from build123d import *

# Parameters (mm, degrees)
PAD_DEPTH           = 2
PAD001_DEPTH        = 3
PAD002_DEPTH        = 3.6
PAD003_DEPTH        = 5
SKETCH004_W         = 63
SKETCH004_H         = 17.5
POCKET_DEPTH        = 11.7
PAD004_DEPTH        = 18
HOLE_D              = 3.3
HOLE_DEPTH          = 24.00858
HOLE_CSINK_D        = 6
HOLE_CSINK_ANGLE    = 90
HOLE_TIPS_R         = 1.65
SKETCH010_R         = 1.75
POCKET001_DEPTH     = 5
HOLE001_D           = 3.3
HOLE001_DEPTH       = 24.00858
HOLE001_CSINK_D     = 6
HOLE001_CSINK_ANGLE = 90
HOLE001_TIPS_R      = 1.65
HOLE002_D           = 3.3
HOLE002_DEPTH       = 24.00858
HOLE002_CSINK_D     = 6
HOLE002_CSINK_ANGLE = 90
HOLE002_TIPS_R      = 1.65


with BuildPart() as part:
    # Sketch → Pad (new body)
    with BuildSketch(Plane.XY):
        Polygon((-31.5, 17.5), (31.5, 17.5), (31.5, -17.5), (15.54, -17.5), (15.54, 2.8e-05), (7.77, 13.458035), (-7.77, 13.458035), (-15.54, 0), (-15.54, -17.5), (-31.5, -17.5), align=None)
    extrude(amount=PAD_DEPTH)

    # Sketch001 (on Face12 of Pad) → Pad001 (join)
    with BuildSketch(Plane.XY.offset(2)):
        with BuildLine():
            ThreePointArc((10, 2.8e-05), (-1.4e-05, 10), (-10, 0))
            Line((-15.54, 0), (-10, 0))
            Line((-15.54, -17.5), (-15.54, 0))
            Line((-15.54, -17.5), (-31.5, -17.5))
            Line((-31.5, -17.5), (-31.5, 17.5))
            Line((-31.5, 17.5), (31.5, 17.5))
            Line((31.5, 17.5), (31.5, -17.5))
            Line((31.5, -17.5), (15.54, -17.5))
            Line((15.54, -17.5), (15.54, 2.8e-05))
            Line((10, 2.8e-05), (15.54, 2.8e-05))
        make_face()
    extrude(amount=PAD001_DEPTH)

    # Sketch002 (on Face20 of Pad001) → Pad002 (join)
    with BuildSketch(Plane.XY.offset(5)):
        Polygon((15.54, 0), (7.77, 13.458035), (-7.77, 13.458035), (-15.54, 0), (-15.54, -17.5), (-31.5, -17.5), (-31.5, 17.5), (31.5, 17.5), (31.5, -17.5), (15.54, -17.5), align=None)
    extrude(amount=PAD002_DEPTH)

    # Sketch003 (on Face31 of Pad002) → Pad003 (join)
    with BuildSketch(Plane.XY.offset(8.6)):
        with BuildLine():
            Line((-31.5, 17.5), (31.5, 17.5))
            Line((31.5, 17.5), (31.5, -17.5))
            Line((31.5, -17.5), (15.54, -17.5))
            Line((15.54, 0), (15.54, -17.5))
            Line((13, 0), (15.54, 0))
            ThreePointArc((13, 0), (0, 13), (-13, 0))
            Line((-15.54, 0), (-13, 0))
            Line((-15.54, 0), (-15.54, -17.5))
            Line((-15.54, -17.5), (-31.5, -17.5))
            Line((-31.5, -17.5), (-31.5, 17.5))
        make_face()
    extrude(amount=PAD003_DEPTH)

    # Sketch004 (on Face41 of Pad003) → Pocket (cut)
    with BuildSketch(Plane.XY.offset(13.6)):
        with Locations((0, -8.75)):
            Rectangle(SKETCH004_W, SKETCH004_H)
    extrude(amount=-POCKET_DEPTH, mode=Mode.SUBTRACT)

    # Sketch008 (on Face1 of Pocket) → Pad004 (join)
    with BuildSketch(Plane(origin=(0, 0, 0), x_dir=(1, 0, 0), z_dir=(0, 0, -1))):
        Polygon((-7.77, -13.458035), (7.77, -13.458035), (15.54, -2.8e-05), (18.54, 0), (8.23, -17.5), (-7.77, -17.5), (-18.54, 0), (-15.54, 0), align=None)
    extrude(amount=PAD004_DEPTH)

    # Hole
    with Locations(Plane(origin=(0, 17.5, 0), x_dir=(-1, 0, 0), z_dir=(0, 1, 0))):
        with Locations((0, -2.45), (-4.5, -10.45), (4.5, -10.45)):
            CounterSinkHole(HOLE_D / 2, HOLE_CSINK_D / 2, depth=HOLE_DEPTH, counter_sink_angle=HOLE_CSINK_ANGLE)

    # Hole tips → Hole tip 1 section 0
    with BuildSketch(Plane(origin=(0, -6.50858, 0), x_dir=(-1, 0, 0), z_dir=(0, 1, 0)), mode=Mode.PRIVATE) as hole_tip_1_s0:
        with Locations((0, -2.45)):
            Circle(HOLE_TIPS_R)
    loft([hole_tip_1_s0.sketch, Vertex(0, -7.5, -2.45)], mode=Mode.SUBTRACT)

    # Hole tips → Hole tip 2 section 0
    with BuildSketch(Plane(origin=(0, -6.50858, 0), x_dir=(-1, 0, 0), z_dir=(0, 1, 0)), mode=Mode.PRIVATE) as hole_tip_2_s0:
        with Locations((-4.5, -10.45)):
            Circle(HOLE_TIPS_R)
    loft([hole_tip_2_s0.sketch, Vertex(4.5, -7.5, -10.45)], mode=Mode.SUBTRACT)

    # Hole tips → Hole tip 3 section 0
    with BuildSketch(Plane(origin=(0, -6.50858, 0), x_dir=(-1, 0, 0), z_dir=(0, 1, 0)), mode=Mode.PRIVATE) as hole_tip_3_s0:
        with Locations((4.5, -10.45)):
            Circle(HOLE_TIPS_R)
    loft([hole_tip_3_s0.sketch, Vertex(-4.5, -7.5, -10.45)], mode=Mode.SUBTRACT)

    # Sketch010 (on Face32 of Hole) → Pocket001 (cut)
    with BuildSketch(Plane.XY.offset(1.9)):
        with Locations((-22.54, -10.7)):
            Circle(SKETCH010_R)
        with Locations((22.54, -10.7)):
            Circle(SKETCH010_R)
    extrude(amount=-POCKET001_DEPTH, mode=Mode.SUBTRACT)

    # Hole001
    with Locations(Plane.XY.offset(13.6)):
        with Locations((-22.54, 10.7), (22.54, 10.7)):
            CounterSinkHole(HOLE001_D / 2, HOLE001_CSINK_D / 2, depth=HOLE001_DEPTH, counter_sink_angle=HOLE001_CSINK_ANGLE)

    # Hole001 tips → Hole001 tip 1 section 0
    with BuildSketch(Plane.XY.offset(-10.40858), mode=Mode.PRIVATE) as hole001_tip_1_s0:
        with Locations((-22.54, 10.7)):
            Circle(HOLE001_TIPS_R)
    loft([hole001_tip_1_s0.sketch, Vertex(-22.54, 10.7, -11.4)], mode=Mode.SUBTRACT)

    # Hole001 tips → Hole001 tip 2 section 0
    with BuildSketch(Plane.XY.offset(-10.40858), mode=Mode.PRIVATE) as hole001_tip_2_s0:
        with Locations((22.54, 10.7)):
            Circle(HOLE001_TIPS_R)
    loft([hole001_tip_2_s0.sketch, Vertex(22.54, 10.7, -11.4)], mode=Mode.SUBTRACT)

    # Hole002
    with Locations(Plane(origin=(0, 17.5, 0), x_dir=(-1, 0, 0), z_dir=(0, 1, 0))):
        with Locations((-27.5, 5.7), (27.5, 5.7)):
            CounterSinkHole(HOLE002_D / 2, HOLE002_CSINK_D / 2, depth=HOLE002_DEPTH, counter_sink_angle=HOLE002_CSINK_ANGLE)

    # Hole002 tips → Hole002 tip 1 section 0
    with BuildSketch(Plane(origin=(0, -6.50858, 0), x_dir=(-1, 0, 0), z_dir=(0, 1, 0)), mode=Mode.PRIVATE) as hole002_tip_1_s0:
        with Locations((-27.5, 5.7)):
            Circle(HOLE002_TIPS_R)
    loft([hole002_tip_1_s0.sketch, Vertex(27.5, -7.5, 5.7)], mode=Mode.SUBTRACT)

    # Hole002 tips → Hole002 tip 2 section 0
    with BuildSketch(Plane(origin=(0, -6.50858, 0), x_dir=(-1, 0, 0), z_dir=(0, 1, 0)), mode=Mode.PRIVATE) as hole002_tip_2_s0:
        with Locations((27.5, 5.7)):
            Circle(HOLE002_TIPS_R)
    loft([hole002_tip_2_s0.sketch, Vertex(-27.5, -7.5, 5.7)], mode=Mode.SUBTRACT)


solid = part.part
Input: part model. Units: mm. Frame: model coordinates. A direction names the side the tool comes from. Give positions to 0.01 mm unless a question says otherwise; leave off trailing zeros. Order: outer loops, then holes, each group sorted by start corner. A loop starts at its lowest first (then second) coordinate and runs counter-clockwise, first axis right, second up. Notation, with made-up numbers: (77.5, 39.25) - (92.5, 39.25) arc R22 cw to (92.5, 60.25) - close; hole circle Ø10 at (26, 9.25). An arc over 180 degrees is marked (long way). Answer as a JSON object with one key per item and string values. Group by question number.
Q1. Cut plane B-B, the plane y = -2.5. Output: boundary loops of the cut face in (x, z), then the cut area to 3 significant figures.
Q2. Cut plane C-C, the plane x = -22.54. Output: boundary loops of the cut face in (y, z), then the cut area to 3 significant figures.
Q3. Mould query, pull axis Z, two halves, no side actions, for faces 4 (the face through (0, 15, 13.6)), 5 (the face through (-31.5, 8, 7)), 6 (the face through (0, 13.458, 7)). Classes: pulls with the +Z half, pulls with the -Z half, needs draft (parallel to the pull), parting line crosses it, or undercut.
Q4. Set-up query: faces 1 (the face through (15.54, -9, 1)), 2 (the face through (11.601, 6.823, -7.86)), 3 (the face through (0, 13, 11)). Return all of +Z, -Z, +X, -X, +Y, -Y with unobstructed straight access to the full face (end or side cutting, diameter ignored); none if empty.
Q5. Cut plane A-A, the plane z = 5.7. Output: boundary loops of the cut face in (x, y).
Q6. Line query: probe 1 along Y at (x, z) = (-22.54, 0.5); probe 2 along Z at (x, y) = (-14, 2.5); probe 3 along Y at (x, z) = (22.54, 3.5). Output: solid intervals per line, ascending.
Q7. Cut plane D-D, the plane y = -10.7. Output: boundary loops of the cut face in (x, z).
Q8. First-contact query: pin 1 Ø4 at (x, y) = (-22.54, -10.7) entering from -Z; pin 2 Ø2.5 at (x, z) = (16.5, -7) entering from -Y; pin 3 Ø4 at (x, y) = (0.5, 9.5) entering from -Z; pin 4 Ø13 at (x, z) = (-21.5, 8) entering from -Y. Flat tips, straight axial feed; report the tip coordinate or a pass-through.
Results:
{
 "1": {"outline": "(-31.5, 0) - (-15.54, 0) - (-15.54, 1.9) - (-31.5, 1.9) - close; (15.54, 0) - (31.5, 0) - (31.5, 1.9) - (15.54, 1.9) - close", "area": "60.6 mm^2"},
 "2": {"outline": "(-17.5, 0) - (-12.45, 0) - (-12.45, 1.9) - (-17.5, 1.9) - close; (-8.95, 0) - (9.05, 0) - (9.05, 12.25) - (7.7, 13.6) - (0, 13.6) - (0, 1.9) - (-8.95, 1.9) - close; (12.35, 0) - (17.5, 0) - (17.5, 13.6) - (13.7, 13.6) - (12.35, 12.25) - close", "area": "218 mm^2"},
 "3": {"face 4": "pulls with the +Z half", "face 5": "needs draft", "face 6": "undercut"},
 "4": {"face 1": "+Z, -Z, -Y", "face 2": "-Z, -Y", "face 3": "+Z, -Y"},
 "5": {"outline": "(-31.5, 0) - (-29.15, 0) - (-29.15, 16.15) - (-30.5, 17.5) - (-31.5, 17.5) - close; (-25.85, 0) - (-15.54, 0) - (-7.77, 13.46) - (7.77, 13.46) - (15.54, 0) - (25.85, 0) - (25.85, 16.15) - (24.5, 17.5) - (-24.5, 17.5) - (-25.85, 16.15) - close; (29.15, 0) - (31.5, 0) - (31.5, 17.5) - (30.5, 17.5) - (29.15, 16.15) - close; hole circle Ø3.3 at (-22.54, 10.7); hole circle Ø3.3 at (22.54, 10.7)"},
 "6": {"probe 1": "-17.5 to -12.45, -8.95 to 9.05, 12.35 to 17.5", "probe 2": "2 to 5, 8.6 to 13.6", "probe 3": "0 to 9.05, 12.35 to 17.5"},
 "7": {"outline": "(-31.5, 0) - (-24.29, 0) - (-24.29, 1.9) - (-31.5, 1.9) - close; (-20.79, 0) - (-15.54, 0) - (-15.54, 1.9) - (-20.79, 1.9) - close; (15.54, 0) - (20.79, 0) - (20.79, 1.9) - (15.54, 1.9) - close; (24.29, 0) - (31.5, 0) - (31.5, 1.9) - (24.29, 1.9) - close"},
 "8": {"pin 1": "z = 0", "pin 2": "y = 0", "pin 3": "z = 2", "pin 4": "y = -17.5"}
}
